Geometry check sheet. Reference: drawing and pictorial views, mm from the part's lowest x, y, z. A direction names the side the tool comes from. Round coordinates to 2 decimals unless told otherwise and drop trailing zeros. Write each loop counter-clockwise with the first axis right and the second up, starting at its lowest first coordinate (ties: lowest second). Pieces come first, ordered by that corner, then holes. Notation, with made-up numbers: (-6.75, -21.75) - (26.25, -21.75) arc R17 ccw to (26.25, -17.75) - close; hole circle Ø9 at (13, -14). An arc over 180 degrees is marked (long way). Return JSON: item names as keys, results as strings.
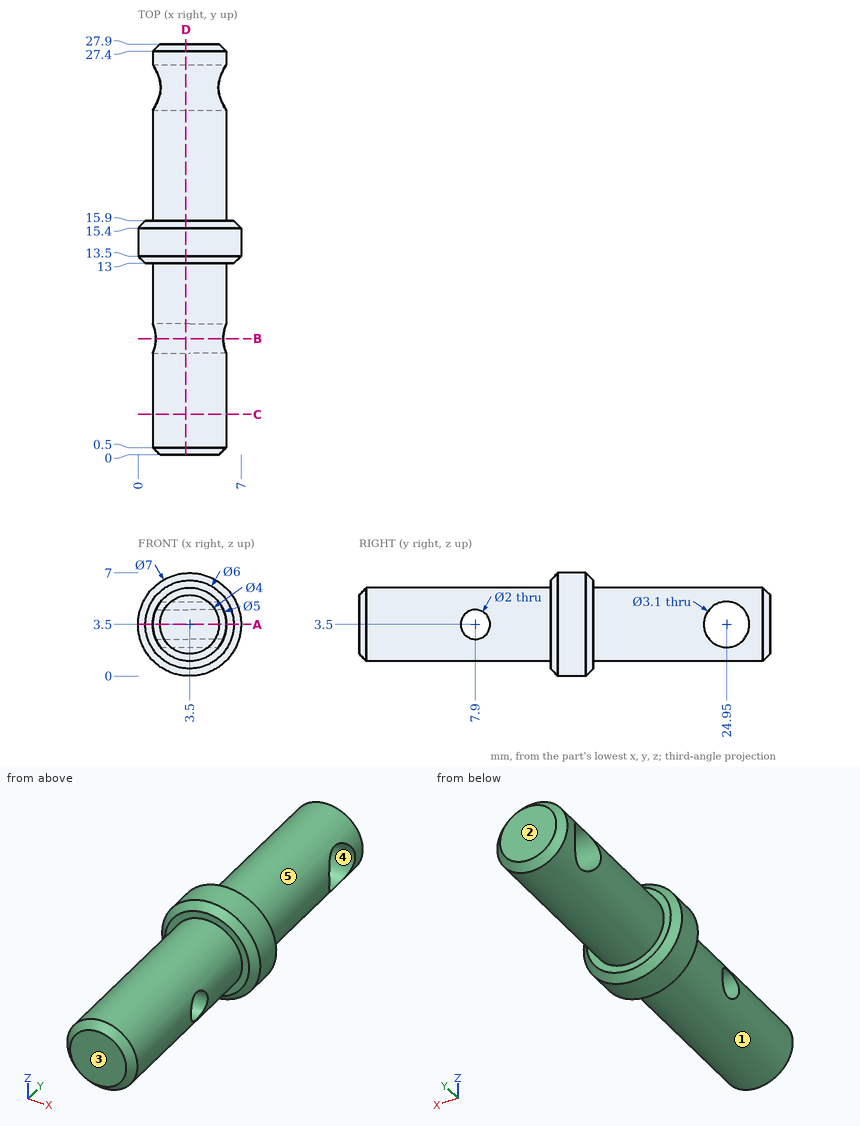
(1) Section check C-C, the plane y = 2.75. Enter the section's corners in (x, z), plus the area to 3 significant figures.
Response values:
{"outline": "circle Ø5 at (3.5, 3.5)", "area": "19.6 mm^2"}
(2) Section check D-D, the plane x = 3.25. Give the number of separate pieces and of enclosed holes in the cut face, plus the area to 3 significant figures.
Response values:
{"separate pieces": "1", "enclosed holes": "2", "area": "133 mm^2"}
(3) Section check B-B, the plane y = 7.9. Enter the section's corners in (x, z), plus the area to 3 significant figures.
Response values:
{"outline": "(1.21, 2.5) arc R2.5 ccw to (5.79, 2.5) - close; (1.21, 4.5) - (5.79, 4.5) arc R2.5 ccw to start", "area": "9.91 mm^2"}
(4) Material ranges on line 1 along Y through (x, z) = (4.95, 3.5); line 2 along Y through (x, z) = (2.25, 3); line 3 along Z through (x, y) = (2, 7.9), recorded low to high. Write a range as [from, to].
Response values:
{"line 1": "y = [0, 6.9], [8.9, 23.4], [26.5, 27.9]", "line 2": "y = [0, 7.03], [8.77, 23.48], [26.42, 27.9]", "line 3": "z = [1.5, 2.5], [4.5, 5.5]"}
(5) Release check for a two-part mould opening along Z. For the marked faces 3, 4 and 5 record: pulls with the +Z half, pulls with the -Z half, needs draft (parallel to the pull), parting line crosses it, or undercut.
Response values:
{"face 3": "needs draft", "face 4": "undercut", "face 5": "parting line crosses it"}
(6) Section check A-A, the plane z = 3.5. Enter the section's corners in (x, y), plus the area to 3 significant figures.
Response values:
{"outline": "(0, 13.5) - (0.5, 13) - (1, 13) - (1, 8.9) - (6, 8.9) - (6, 13) - (6.5, 13) - (7, 13.5) - (7, 15.4) - (6.5, 15.9) - (6, 15.9) - (6, 23.4) - (1, 23.4) - (1, 15.9) - (0.5, 15.9) - (0, 15.4) - close; (1, 0.5) - (1.5, 0) - (5.5, 0) - (6, 0.5) - (6, 6.9) - (1, 6.9) - close; (1, 26.5) - (6, 26.5) - (6, 27.4) - (5.5, 27.9) - (1.5, 27.9) - (1, 27.4) - close", "area": "119 mm^2"}
(7) Gauge pin test, flat ends, axial feed: pin 1 (3.5 mm diameter, centred on y = 24.95, z = 3.5, fed in from -X); pin 2 (2 mm diameter, centred on x = 6, y = 23, fed in from -Z); pin 3 (1.8 mm diameter, centred on y = 7.9, z = 3.5, fed in from -X). Record the tip position at first contact, or that the pin passes through.
Response values:
{"pin 1": "stops at x = 1", "pin 2": "stops at z = 1.5", "pin 3": "passes through"}
(8) Access from +Z, -Z, +X, -X, +Y, -Y to the whole of each face (thin tool, end or side, straight path). Record for the marked faces 1 and 2.
Response values:
{"face 1": "-Y", "face 2": "+Z, -Z, +X, -X, +Y"}
